Check sheet for the drawn part. Datum: minimum x, y, z corner. Units: mm. A direction names the side the tool comes from. Give positions to 0.01 mm unless a question says otherwise; leave off trailing zeros. Loops run counter-clockwise (first coordinate to the right, second up) from the corner with the lowest first, then second, coordinate; pieces in that order, holes last. Notation, with made-up numbers: (1, -9) - (60, -9) arc R23 cw to (60, 7) - close; hole circle Ø11 at (-35, 57). An arc over 180 degrees is marked (long way). Use one line per item in the form item = value.
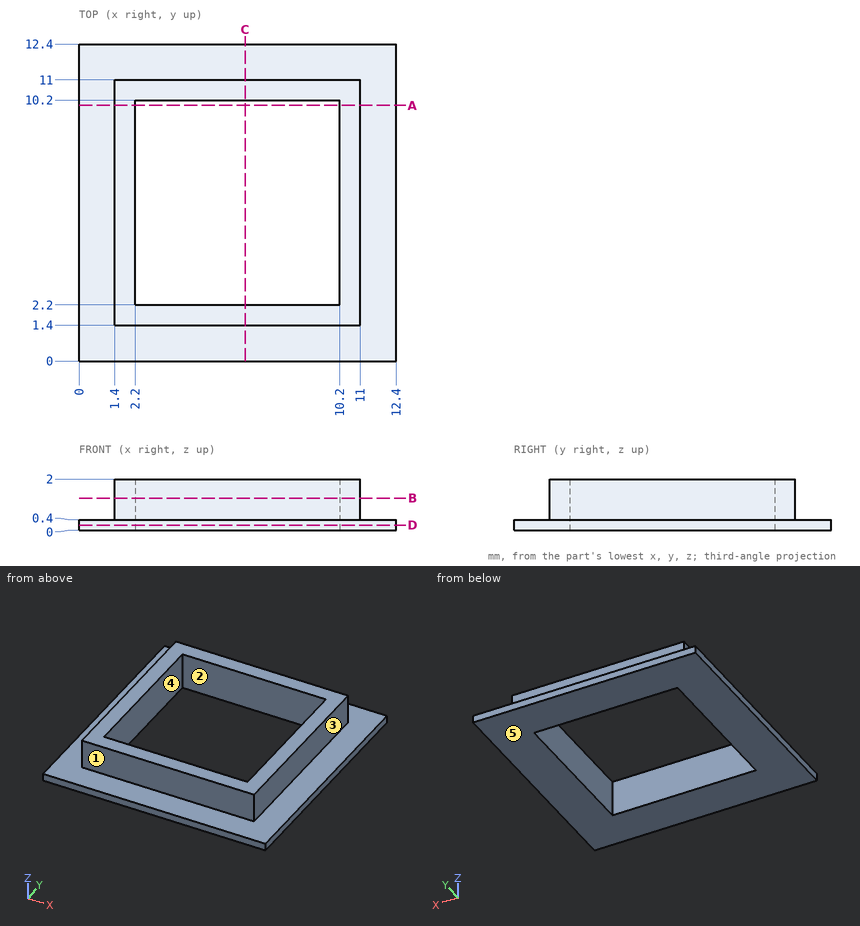
Item 1: Thickness scan on L1, parallel to X at y = 4.25, z = 0.9; L2, parallel to X at y = 6.25, z = 0.25. Record the ranges inside material, lowest first.
Answer block:
L1 = 1.4 to 2.2, 10.2 to 11
L2 = 0 to 2.2, 10.2 to 12.4
Item 2: Section check D-D on z = 0.2. Record the boundary of the cut face in (x, y).
Answer block:
outline = (0, 0) - (12.4, 0) - (12.4, 12.4) - (0, 12.4) - close; hole (2.2, 2.2) - (10.2, 2.2) - (10.2, 10.2) - (2.2, 10.2) - close
Item 3: Gauge pin test, flat ends, axial feed: P1, Ø0.5, axis at x = 7.5, z = 1, coming from the +Y side; P2, Ø0.5, axis at y = 6, z = 1.5, coming from the -X side; P3, Ø1, axis at x = 10.5, z = 1, coming from the -Y side. Record the tip position at first contact, or that the pin passes through.
Answer block:
P1 = 11
P2 = 1.4
P3 = 1.4
Item 4: Access from +Z, -Z, +X, -X, +Y, -Y to the whole of each face (thin tool, end or side, straight path). Record for the marked faces 1 and 2.
Answer block:
face_1 = +Z, +X, -X, -Y
face_2 = +Z, -Z
Item 5: Section check B-B on z = 1.25. Record the boundary of the cut face in (x, y).
Answer block:
outline = (1.4, 1.4) - (11, 1.4) - (11, 11) - (1.4, 11) - close; hole (2.2, 2.2) - (10.2, 2.2) - (10.2, 10.2) - (2.2, 10.2) - close
Item 6: Mould release check, pull along X, two halves, no side actions. Record for the marked faces 3, 4 and 5: released by +X, released by -X, zero draft, split by the parting line, or undercut.
Answer block:
face_3 = released by +X
face_4 = undercut
face_5 = zero draft
Item 7: Section check A-A on y = 10. Record the boundary of the cut face in (x, z).
Answer block:
outline = (0, 0) - (2.2, 0) - (2.2, 2) - (1.4, 2) - (1.4, 0.4) - (0, 0.4) - close; (10.2, 0) - (12.4, 0) - (12.4, 0.4) - (11, 0.4) - (11, 2) - (10.2, 2) - close
